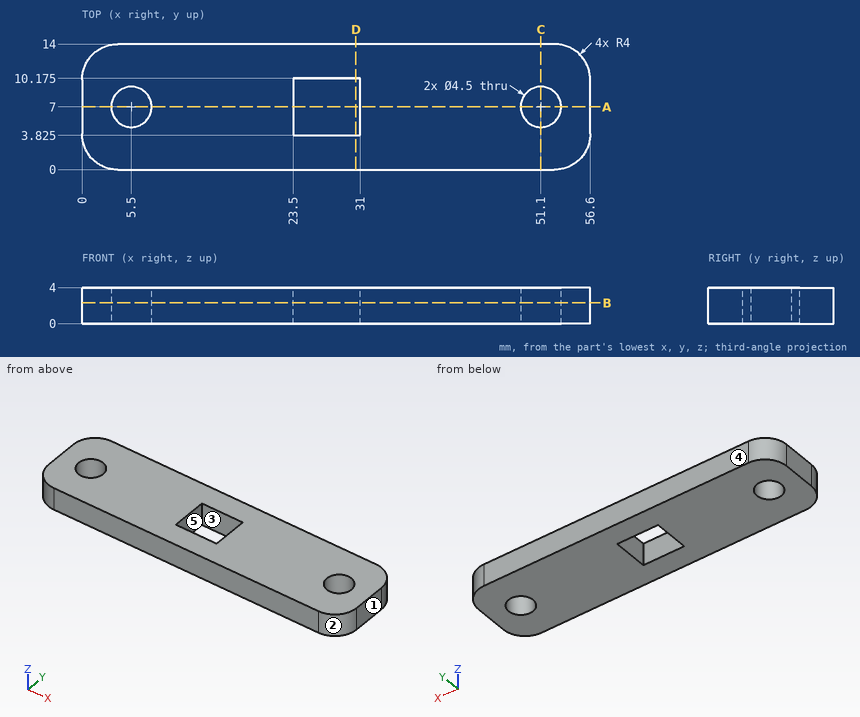
Geometry check sheet. Reference: drawing and pictorial views, mm from the part's lowest x, y, z. A direction names the side the tool comes from. Give positions to 0.01 mm unless a question says otherwise; leave off trailing zeros. Order: outer loops, then holes, each group sorted by start corner. A loop starts at its lowest first (then second) coordinate and runs counter-clockwise, first axis right, second up. Notation, with made-up numbers: (23, 37) -> (52, 37) arc R28 cw to (52, 60) -> close; hole circle Ø11 at (77.5, -11). An arc over 180 degrees is marked (long way). Use CSV: the item, a comma, the result in double quotes. Start each with the question number.
1) Set-up check for the marked faces 4 and 5: record each of +Z, -Z, +X, -X, +Y, -Y from which the full face is reachable in a straight line by a thin tool's end or side.
2) Sectioned sample at B-B, the plane z = 2.3. Record the boundary of the cut face in (x, y) (3 decimals), plus the area to 3 significant figures.
3) Sectioned sample at C-C, the plane x = 51.1. Record the boundary of the cut face in (y, z).
4) Sectioned sample at A-A, the plane y = 7. Record the boundary of the cut face in (x, z).
5) Mould release check, pull along Y, two halves, no side actions. Record for the marked faces 1, 2 and 3: released by +Y, released by -Y, zero draft, split by the parting line, or undercut.
6) Sectioned sample at D-D, the plane x = 30.5. Record the boundary of the cut face in (y, z) (3 decimals), plus the area to 3 significant figures.
7) Material ranges on line 1 (Y direction, x = 5.5, z = 3); line 2 (Y direction, x = 27.5, z = 2.1) (3 decimals); line 3 (X direction, y = 4.25, z = 2.55), recorded low to high. Write a range as from..to.
Recorded:
1,face 4,"+Z, -Z, +X, -X, +Y"
1,face 5,"+Z, -Z"
2,outline,"(0, 4) arc R4 ccw to (4, 0) -> (52.6, 0) arc R4 ccw to (56.6, 4) -> (56.6, 10) arc R4 ccw to (52.6, 14) -> (4, 14) arc R4 ccw to (0, 10) -> close; hole circle Ø4.5 at (5.5, 7); hole (23.5, 3.825) -> (31, 3.825) -> (31, 10.175) -> (23.5, 10.175) -> close; hole circle Ø4.5 at (51.1, 7)"
2,area,"699 mm2"
3,outline,"(0, 0) -> (4.75, 0) -> (4.75, 4) -> (0, 4) -> close; (9.25, 0) -> (14, 0) -> (14, 4) -> (9.25, 4) -> close"
4,outline,"(0, 0) -> (3.25, 0) -> (3.25, 4) -> (0, 4) -> close; (7.75, 0) -> (23.5, 0) -> (23.5, 4) -> (7.75, 4) -> close; (31, 0) -> (48.85, 0) -> (48.85, 4) -> (31, 4) -> close; (53.35, 0) -> (56.6, 0) -> (56.6, 4) -> (53.35, 4) -> close"
5,face 1,"zero draft"
5,face 2,"released by -Y"
5,face 3,"undercut"
6,outline,"(0, 0) -> (3.825, 0) -> (3.825, 4) -> (0, 4) -> close; (10.175, 0) -> (14, 0) -> (14, 4) -> (10.175, 4) -> close"
6,area,"30.6 mm2"
7,line 1,"0..4.75, 9.25..14"
7,line 2,"0..3.825, 10.175..14"
7,line 3,"0..23.5, 31..56.6"
